```python
from build123d import *

# Parameters (mm, degrees)
SKETCH1_R           = 7
SKETCH1_R_2         = 3.5
BOSS_EXTRUDE1_DEPTH = 7
SKETCH2_R           = 12.25
BOSS_EXTRUDE2_DEPTH = 4.2
CUT_EXTRUDE1_START  = -2.1
CUT_EXTRUDE1_DEPTH  = 2.1
CUT_EXTRUDE2_START  = -2.1
SKETCH4_R           = 3.5
CUT_EXTRUDE2_DEPTH  = 2.1


with BuildPart() as part:
    # Sketch1 → Boss-Extrude1 (new body)
    with BuildSketch(Plane.XY):
        Circle(SKETCH1_R)
        Circle(SKETCH1_R_2, mode=Mode.SUBTRACT)
    extrude(amount=BOSS_EXTRUDE1_DEPTH)

    # Sketch2 → Boss-Extrude2 (add)
    with BuildSketch(Plane(origin=(0, 0, 0), x_dir=(-1, 0, 0), z_dir=(0, 0, -1))):
        Circle(SKETCH2_R)
    extrude(amount=BOSS_EXTRUDE2_DEPTH)

    # Sketch3 → Cut-Extrude1 (cut)
    with BuildSketch(Plane(origin=(0, 0, -4.2), x_dir=(-1, 0, 0), z_dir=(0, 0, -1)).offset(CUT_EXTRUDE1_START)):
        with BuildLine():
            Line((-12.124355653, 1.75), (12.124355653, 1.75))
            ThreePointArc((12.124355653, 1.75), (12.25, 0), (12.124355653, -1.75))
            Line((12.124355653, -1.75), (-12.124355653, -1.75))
            ThreePointArc((-12.124355653, -1.75), (-12.25, 0), (-12.124355653, 1.75))
        make_face()
    extrude(amount=CUT_EXTRUDE1_DEPTH, mode=Mode.SUBTRACT)

    # Sketch4 → Cut-Extrude2 (cut)
    with BuildSketch(Plane.XY.offset(CUT_EXTRUDE2_START)):
        with Locations(Location((0, 0, 0), (0, 0, 210))):
            Circle(SKETCH4_R)
    extrude(amount=CUT_EXTRUDE2_DEPTH, mode=Mode.SUBTRACT)


solid = part.part
```
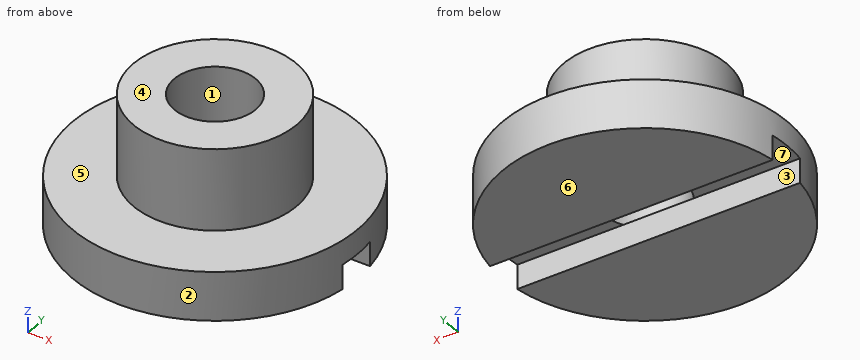
Design review of the part built by this model. Coordinates are the model's own, in mm. Face numbers are marked on the shaded views. A direction names the side the tool comes from. Coordinates: 2 decimals unless noted, no trailing zeros. Order: outer loops, then holes, each group sorted by start corner. A loop starts at its lowest first (then second) coordinate and runs counter-clockwise, first axis right, second up. Notation, with made-up numbers: M 25.25,-11.75 L 46.25,-11.75 A7 cw 46.25,-2.75 Z; hole C 36.5,66.25 d10. An arc over 180 degrees is marked long. Answer as a JSON object with one key per item and string values. Group by question number.
1) Mouldability with a two-part tool opening along Y and no side actions: class the marked faces 1, 2, 3 and 4 as pulls with the +Y half, pulls with the -Y half, needs draft (parallel to the pull), parting line crosses it, or undercut.
2) Wall thickness on L1, parallel to Y at x = 0, z = 4.25; L2, parallel to Z at x = 4, y = 0.5; L3, parallel to Y at x = -9.5, z = -2.25: over which ranges is each line inside the solid? List them lowest first.
3) Add section C-C, the plane z = 3. Write out the cut boundary in (x, y).
4) Tool access review of the marked faces 5, 6 and 7: name each direction out of +Z, -Z, +X, -X, +Y, -Y from which nothing blocks a thin tool from reaching the whole face with its end or side.
5) Add section A-A, the plane x = 0. Write out the cut boundary in (y, z), then the cut area to 3 significant figures.
6) Add section D-D, the plane x = -9.5. Write out the cut boundary in (y, z).
7) For pin 1 (1 mm diameter, centred on x = 4, z = -2.5, fed in from -Y); pin 2 (5 mm diameter, centred on x = -7, z = -2, fed in from -Y); pin 3 (6 mm diameter, centred on x = 4, z = 4.5, fed in from +Y), all flat-tipped, find the tip position at first contact; note any pin that passes through.
8) Add section B-B, the plane y = 0. Write out the cut boundary in (x, z), then the cut area to 4 significant figures.
Computed values:
{
 "1": {"face 1": "undercut", "face 2": "parting line crosses it", "face 3": "undercut", "face 4": "needs draft"},
 "2": {"L1": "y = -7 to -3.5, 3.5 to 7", "L2": "z = -2.1 to 7", "L3": "y = -7.73 to -1.75, 1.75 to 7.73"},
 "3": {"outline": "C 0,0 d14; hole C 0,0 d7"},
 "4": {"face 5": "+Z", "face 6": "-Z, +X, -X, +Y, -Y", "face 7": "-Z, +X, -X"},
 "5": {"outline": "M -12.25,-4.2 L -1.75,-4.2 L -1.75,-2.1 L -3.5,-2.1 L -3.5,7 L -7,7 L -7,0 L -12.25,0 Z; M 1.75,-4.2 L 12.25,-4.2 L 12.25,0 L 7,0 L 7,7 L 3.5,7 L 3.5,-2.1 L 1.75,-2.1 Z", "area": "130 mm^2"},
 "6": {"outline": "M -7.73,-4.2 L -1.75,-4.2 L -1.75,-2.1 L 1.75,-2.1 L 1.75,-4.2 L 7.73,-4.2 L 7.73,0 L -7.73,0 Z"},
 "7": {"pin 1": "stops at y = -11.74", "pin 2": "stops at y = -11.39", "pin 3": "stops at y = 6.93"},
 "8": {"outline": "M -12.25,-2.1 L -3.5,-2.1 L -3.5,7 L -7,7 L -7,0 L -12.25,0 Z; M 3.5,-2.1 L 12.25,-2.1 L 12.25,0 L 7,0 L 7,7 L 3.5,7 Z", "area": "85.75 mm^2"}
}
